Read the model definition and answer for the solid it produces. Units are mm, in the model's axes. Face numbers are marked on the shaded views. A direction names the side the tool comes from. Round coordinates to 2 decimals unless told otherwise and drop trailing zeros. Write each loop counter-clockwise with the first axis right and the second up, starting at its lowest first coordinate (ties: lowest second). Pieces come first, ordered by that corner, then holes.
from build123d import *

# Parameters (mm, degrees)
SKETCH1_W           = 40
SKETCH1_H           = 10
BOSS_EXTRUDE1_DEPTH = 36
CUT_EXTRUDE1_DEPTH  = 10
SKETCH3_R           = 2.6
CUT_EXTRUDE2_DEPTH  = 55.735728734
BOSS_EXTRUDE2_START = 4.2
SKETCH5_R           = 2.6
BOSS_EXTRUDE2_DEPTH = 4.2


with BuildPart() as part:
    # Sketch1 → Boss-Extrude1 (new, symmetric)
    with BuildSketch(Plane(origin=(0, 0, 0), x_dir=(1, 0, 0), z_dir=(0, 1, 0))):
        with Locations((20, 5)):
            Rectangle(SKETCH1_W, SKETCH1_H)
    extrude(amount=BOSS_EXTRUDE1_DEPTH, both=True)

    # Sketch2 → Cut-Extrude1 (cut)
    with BuildSketch(Plane(origin=(40, 0, 0), x_dir=(0, 0, -1), z_dir=(1, 0, 0))):
        with BuildLine():
            Line((0, 26.35), (0, 13.65))
            ThreePointArc((0, 13.65), (6.35, 20), (0, 26.35))
        make_face()
        with BuildLine():
            Line((0, -13.65), (0, -26.35))
            ThreePointArc((0, -26.35), (6.35, -20), (0, -13.65))
        make_face()
    extrude(amount=-CUT_EXTRUDE1_DEPTH, mode=Mode.SUBTRACT)

    # Sketch3 → Cut-Extrude2 (cut, through all)
    with BuildSketch(Plane(origin=(0, 0, -10), x_dir=(-1, 0, 0), z_dir=(0, 0, -1))):
        with Locations((-35, 31)):
            Circle(SKETCH3_R)
        with Locations((-5, 31)):
            Circle(SKETCH3_R)
        with Locations((-35, -31)):
            Circle(SKETCH3_R)
        with Locations((-5, -31)):
            Circle(SKETCH3_R)
        with Locations((-35, 0)):
            Circle(SKETCH3_R)
    extrude(amount=-CUT_EXTRUDE2_DEPTH, mode=Mode.SUBTRACT)

    # Sketch5 → Boss-Extrude2 (add)
    with BuildSketch(Plane(origin=(0, 0, -10), x_dir=(-1, 0, 0), z_dir=(0, 0, -1)).offset(BOSS_EXTRUDE2_START)):
        with BuildLine():
            Line((-40, 8.660254038), (-40, -8.660254038))
            ThreePointArc((-40, -8.660254038), (-25, 0), (-40, 8.660254038))
        make_face()
        with Locations((-35, 0)):
            Circle(SKETCH5_R, mode=Mode.SUBTRACT)
    extrude(amount=-BOSS_EXTRUDE2_DEPTH)


solid = part.part
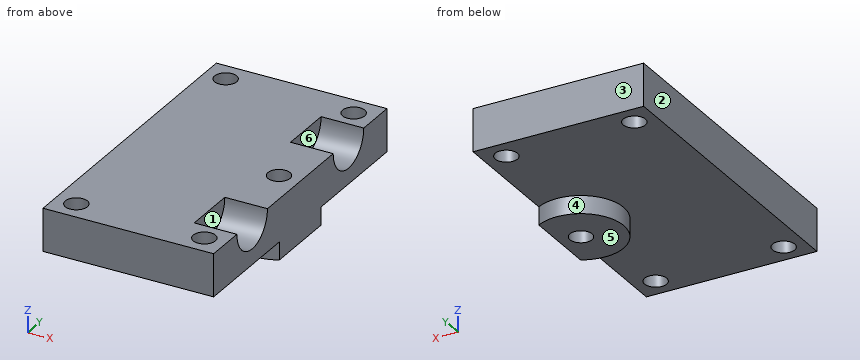
Q1. Determine the mould class of the marked faces 1, 2 and 3 for opening direction Y: pulls with the +Y half, pulls with the -Y half, needs draft (parallel to the pull), parting line crosses it, or undercut.
Verdict:
face 1: undercut
face 2: needs draft
face 3: pulls with the +Y half
Q2. Section A-A (y = 31) is taken. Determine the outline of the cut face in (x, z), then the cut area to 3 significant figures.
Verdict:
outline: (0, -10) - (2.4, -10) - (2.4, 0) - (0, 0) - close; (7.6, -10) - (32.4, -10) - (32.4, 0) - (7.6, 0) - close; (37.6, -10) - (40, -10) - (40, 0) - (37.6, 0) - close
area: 296 mm2
Q3. Straight lines are drawn through the part: probe 1 along Y at (x, z) = (5, -6.25); probe 2 along X at (y, z) = (-30.5, -4.75); probe 3 along Z at (x, y) = (14.5, 9.5). For each, find the intervals that lie inside material, in ascending order.
Verdict:
probe 1: y = -36 to -33.6, -28.4 to 28.4, 33.6 to 36
probe 2: x = 0 to 2.45, 7.55 to 32.45, 37.55 to 40
probe 3: z = -10 to 0
Q4. Section D-D (z = -7.5) is taken. Determine the outline of the cut face in (x, y).
Verdict:
outline: (0, -36) - (40, -36) - (40, 36) - (0, 36) - close; hole circle Ø5.2 at (5, -31); hole circle Ø5.2 at (5, 31); hole circle Ø5.2 at (35, -31); hole circle Ø5.2 at (35, 0); hole circle Ø5.2 at (35, 31)
Q5. Section C-C (x = 5) is taken. Determine the outline of the cut face in (y, z), then the cut area to 3 significant figures.
Verdict:
outline: (-36, -10) - (-33.6, -10) - (-33.6, 0) - (-36, 0) - close; (-28.4, -10) - (28.4, -10) - (28.4, 0) - (-28.4, 0) - close; (33.6, -10) - (36, -10) - (36, 0) - (33.6, 0) - close
area: 616 mm2
Q6. Which of the six approach directions +Z, -Z, +X, -X, +Y, -Y give full straight-line access (tool end or side, diameter ignored) to the marked faces 4, 5 and 6?
Verdict:
face 4: -Z
face 5: -Z, +X, -X, +Y, -Y
face 6: +Z, +X
Q7. Flat-ended cylindrical pins translate along their axes: pin 1 Ø1.9 at (y, z) = (-23, -3) entering from +X; pin 2 Ø4 at (x, y) = (29.5, -21) entering from -Z; pin 3 Ø4.5 at (x, y) = (5, 31) entering from -Z. Find the tip coordinate at first contact, or state that the pin passes through.
Verdict:
pin 1: stops at x = 30
pin 2: stops at z = -10
pin 3: passes through
Q8. Section B-B (x = 35) is taken. Determine the outline of the cut face in (y, z).
Verdict:
outline: (-36, -10) - (-33.6, -10) - (-33.6, 0) - (-36, 0) - close; (-28.4, -10) - (-10, -10) - (-10, -14.2) - (-2.6, -14.2) - (-2.6, 0) - (-13.65, 0) arc R6.35 cw to (-26.35, 0) - (-28.4, 0) - close; (2.6, -14.2) - (10, -14.2) - (10, -10) - (28.4, -10) - (28.4, 0) - (26.35, 0) arc R6.35 cw to (13.65, 0) - (2.6, 0) - close; (33.6, -10) - (36, -10) - (36, 0) - (33.6, 0) - close
